from build123d import *

# Parameters (mm, degrees)
BODY_DEPTH                = 6
SKETCH2_W                 = 19.1
SKETCH2_H                 = 6
TOP_TAB_DEPTH             = 6
SKETCH3_W                 = 6
SKETCH3_H                 = 5.5
BACK_TAB_DEPTH            = 6
SKETCH5_R                 = 1.7
BACK_SCREW_HOLE_DEPTH     = 12
SCREW_AND_NUT_HOLES_REACH = 8
SKETCH4_R                 = 1.7
SKETCH4_W                 = 2.5
SKETCH4_H                 = 6
SKETCH7_R                 = 3.5
SWITCH_WIRE_RELIEF_DEPTH  = 7
FILLET1_R                 = 0.5
SERVO_OPENINGS_REACH      = 8
SKETCH6_R                 = 0.75
CHAMFER1_SIZE             = 0.5
SKETCH8_W                 = 2
SKETCH8_H                 = 3
CUT_EXTRUDE1_DEPTH        = 7.0000001


with BuildPart() as part:
    # Sketch1 → Body (new body)
    with BuildSketch(Plane.XY):
        Polygon((0, -26.5), (15, -26.5), (47, -17), (47, 0), (0, 0), align=None)
    extrude(amount=-BODY_DEPTH)

    # Sketch2 → Top Tab (add)
    with BuildSketch(Plane(origin=(0, 0, 0), x_dir=(1, 0, 0), z_dir=(0, 1, 0))):
        with Locations((22.5, 3)):
            Rectangle(SKETCH2_W, SKETCH2_H)
    extrude(amount=TOP_TAB_DEPTH)

    # Sketch3 → Back Tab (add)
    with BuildSketch(Plane.ZY):
        with Locations((-3, -18.69)):
            Rectangle(SKETCH3_W, SKETCH3_H)
    extrude(amount=BACK_TAB_DEPTH)

    # Sketch5 → Back Screw Hole (cut)
    with BuildSketch(Plane.ZY):
        with Locations((-3, -11)):
            Circle(SKETCH5_R)
    extrude(amount=-BACK_SCREW_HOLE_DEPTH, mode=Mode.SUBTRACT)

    # Sketch4 → Screw and Nut Holes (cut, up to next)
    with BuildSketch(Plane.XY, mode=Mode.PRIVATE) as screw_and_nut_holes_sk1:
        with Locations((22.5, 3)):
            Circle(SKETCH4_R)
    screw_and_nut_holes_tool1 = extrude(screw_and_nut_holes_sk1.sketch, amount=-SCREW_AND_NUT_HOLES_REACH, mode=Mode.PRIVATE) & part.part
    add(screw_and_nut_holes_tool1.solids().sort_by_distance((22.5, 3, 0))[0], mode=Mode.SUBTRACT)
    # Sketch4 → Screw and Nut Holes (cut, up to next)
    with BuildSketch(Plane.XY, mode=Mode.PRIVATE) as screw_and_nut_holes_sk2:
        with Locations((8.25, -11)):
            Rectangle(SKETCH4_W, SKETCH4_H)
    screw_and_nut_holes_tool2 = extrude(screw_and_nut_holes_sk2.sketch, amount=-SCREW_AND_NUT_HOLES_REACH, mode=Mode.PRIVATE) & part.part
    add(screw_and_nut_holes_tool2.solids().sort_by_distance((8.25, -11, 0))[0], mode=Mode.SUBTRACT)

    # Sketch7 → Switch Wire Relief (cut, through all)
    with BuildSketch(Plane.XY):
        Circle(SKETCH7_R)
    extrude(amount=-SWITCH_WIRE_RELIEF_DEPTH, mode=Mode.SUBTRACT)

    # Fillet1
    fillet1_edges = [part.edges().sort_by_distance(p)[0] for p in [
        (32.05, 6, -3),
        (12.95, 6, -3),
        (-6, -15.94, -3),
        (-6, -21.44, -3),
        (7.5, -26.5, -6),
        (31, -21.75, -6),
        (47, -8.5, -6),
        (39.525, 0, -6),
        (32.05, 3, -6),
        (22.5, 6, -6),
        (12.95, 3, -6),
        (8.225, 0, -6),
        (0, -9.72, -6),
        (-3, -15.94, -6),
        (-6, -18.69, -6),
        (-3, -21.44, -6),
        (0, -23.97, -6),
        (0, -9.72, 0),
        (8.225, 0, 0),
        (12.95, 3, 0),
        (22.5, 6, 0),
        (32.05, 3, 0),
        (39.525, 0, 0),
        (47, -8.5, 0),
        (31, -21.75, 0),
        (7.5, -26.5, 0),
        (0, -23.97, 0),
        (-3, -21.44, 0),
        (-6, -18.69, 0),
        (-3, -15.94, 0),
        (2.474873734, -2.474873734, -6),
        (2.474873734, -2.474873734, 0),
    ]]
    fillet(fillet1_edges, radius=FILLET1_R)

    # Sketch6 → Servo Openings (cut, up to next)
    with BuildSketch(Plane.XY, mode=Mode.PRIVATE) as servo_openings_sk1:
        with Locations((14.056274553, -16.473540836)):
            Circle(SKETCH6_R)
    servo_openings_tool1 = extrude(servo_openings_sk1.sketch, amount=-SERVO_OPENINGS_REACH, mode=Mode.PRIVATE) & part.part
    add(servo_openings_tool1.solids().sort_by_distance((14.056275, -16.473541, 0))[0], mode=Mode.SUBTRACT)
    # Sketch6 → Servo Openings (cut, up to next)
    with BuildSketch(Plane.XY, mode=Mode.PRIVATE) as servo_openings_sk2:
        with Locations((40.323198689, -8.675547733)):
            Circle(SKETCH6_R)
    servo_openings_tool2 = extrude(servo_openings_sk2.sketch, amount=-SERVO_OPENINGS_REACH, mode=Mode.PRIVATE) & part.part
    add(servo_openings_tool2.solids().sort_by_distance((40.323199, -8.675548, 0))[0], mode=Mode.SUBTRACT)
    # Sketch6 → Servo Openings (cut, up to next)
    with BuildSketch(Plane.XY, mode=Mode.PRIVATE) as servo_openings_sk3:
        Polygon((36.401733852, -3.372283311), (39.930752628, -15.259504453), (17.97773939, -21.776805258), (14.448720614, -9.889584116), align=None)
    servo_openings_tool3 = extrude(servo_openings_sk3.sketch, amount=-SERVO_OPENINGS_REACH, mode=Mode.PRIVATE) & part.part
    add(servo_openings_tool3.solids().sort_by_distance((27.189737, -12.574544, 0))[0], mode=Mode.SUBTRACT)

    # Chamfer1
    chamfer1_edges = [part.edges().sort_by_distance(p)[0] for p in [
        (25.425227233, -6.630933714, 0),
        (16.213230002, -15.833194687, 0),
        (28.954246009, -18.518154856, 0),
        (38.16624324, -9.315893882, 0),
        (16.213230002, -15.833194687, -6),
        (25.425227233, -6.630933714, -6),
        (38.16624324, -9.315893882, -6),
        (28.954246009, -18.518154856, -6),
        (13.306274553, -16.473540836, 0),
        (13.306274553, -16.473540836, -6),
        (39.573198689, -8.675547733, 0),
        (39.573198689, -8.675547733, -6),
    ]]
    chamfer(chamfer1_edges, length=CHAMFER1_SIZE)

    # Sketch8 → Cut-Extrude1 (cut, through all)
    with BuildSketch(Plane.XY):
        with Locations((44, -6.5)):
            Rectangle(SKETCH8_W, SKETCH8_H)
    extrude(amount=-CUT_EXTRUDE1_DEPTH, mode=Mode.SUBTRACT)


solid = part.part
The listing builds one solid part. Answer for the finished solid, in the listing's coordinates (mm). A direction names the side the tool comes from. Round coordinates to 2 decimals unless told otherwise and drop trailing zeros. Write each loop counter-clockwise with the first axis right and the second up, starting at its lowest first coordinate (ties: lowest second). Pieces come first, ordered by that corner, then holes. Notation, with made-up numbers: M -0.5,79.5 L 11.5,79.5 A15 cw 11.5,88.5 Z; hole C -14.75,43 d3. An arc over 180 degrees is marked long. Write each question's results on one line, items separated by ' | '. Start each with the question number.
(1) For faces 1 (the flat face through (40, 0, -3)), 2 (the flat face through (45, -7, -3)), 3 (the flat face through (-3, -21.44, -3)), determine the directions among +Z, -Z, +X, -X, +Y, -Y from which every point of the face is accessible in a straight line to the end or side of a thin tool.
(2) The part is cut by section C-C, the plane y = -11. Write down the section's boundary in (x, z), and give its area (3 significant figures).
(3) The part is cut by section B-B, the plane x = -2. Write down the section's boundary in (y, z), and give its area (3 significant figures).
(4) The part is cut by section A-A, the plane y = 3. Write down the section's boundary in (x, z).
(5) Find the intervals of material crossed by line 1 (Y direction, x = 11.55, z = -3); line 2 (Y direction, x = 24, z = -2.5); line 3 (Y direction, x = 23, z = -4) (3 decimals), in increasing order.
(6) The part is cut by section D-D, the plane x = 5. Write down the section's boundary in (y, z).
(7) Determine the mould class of faces 4 (the flat face through (-6, -19, -3)), 5 (the flat face through (7, -26.5, -3)), 6 (the flat face through (25.272, -6.677, -2.965)) for opening direction Y: +Y half, -Y half, draft (parallel to the pull), parting line (faces both ways), or undercut.
(8) Each of these flat-tipped pins is pushed along its axis until it touches: P1, Ø3.5, axis at y = -7, z = -3, coming from the -X side; P2, Ø2, axis at x = 43.5, z = -2.5, coming from the +Y side; P3, Ø1.4, axis at x = 14.06, y = -16.47, coming from the -Z side; P4, Ø2.5, axis at y = -11, z = -3, coming from the -X side. Where does it stop, or does it pass through?
Worked answers:
1) face 1: +Z, -Z, +X, +Y | face 2: +Z, -Z | face 3: +Z, -Z, -X, -Y
2) outline: M 0,-5.5 A0.5 ccw 0.5,-6 L 7,-6 L 7,-4.7 L 0,-4.7 Z; M 0,-1.3 L 7,-1.3 L 7,0 L 0.5,0 A0.5 ccw 0,-0.5 Z; M 9.5,-6 L 14.26,-6 L 14.78,-5.5 L 14.78,-0.5 L 14.26,0 L 9.5,0 L 9.5,-1.3 L 12,-1.3 L 12,-4.7 L 9.5,-4.7 Z; M 38.67,-5.5 L 39.19,-6 L 46.5,-6 A0.5 ccw 47,-5.5 L 47,-0.5 A0.5 ccw 46.5,0 L 39.19,0 L 38.67,-0.5 Z | area: 90.6 mm²
3) outline: M -21.44,-5.5 A0.5 ccw -20.94,-6 L -16.44,-6 A0.5 ccw -15.94,-5.5 L -15.94,-0.5 A0.5 ccw -16.44,0 L -20.94,0 A0.5 ccw -21.44,-0.5 Z | area: 32.8 mm²
4) outline: M 12.95,-5.5 A0.5 ccw 13.45,-6 L 20.8,-6 L 20.8,0 L 13.45,0 A0.5 ccw 12.95,-0.5 Z; M 24.2,-6 L 31.55,-6 A0.5 ccw 32.05,-5.5 L 32.05,-0.5 A0.5 ccw 31.55,0 L 24.2,0 Z
5) line 1: y = -26.5 to -12.7, -9.3 to 0 | line 2: y = -23.83 to -19.99, -7.05 to 2.2, 3.8 to 6 | line 3: y = -24.125 to -20.286, -7.351 to 1.375, 4.625 to 6
6) outline: M -26.5,-5.5 A0.5 ccw -26,-6 L -0.5,-6 A0.5 ccw 0,-5.5 L 0,-0.5 A0.5 ccw -0.5,0 L -26,0 A0.5 ccw -26.5,-0.5 Z; hole C -11,-3 d3.4
7) face 4: draft | face 5: -Y half | face 6: undercut
8) P1: stops at x = 0 | P2: stops at y = 0 | P3: passes through | P4: stops at x = 12
